```python
from build123d import *


with BuildPart() as part:
    # Sketch1 → Revolve1 (revolve)
    with BuildSketch(Plane.XY, mode=Mode.PRIVATE) as revolve1_sk:
        with BuildLine():
            Line((-40, 5), (-40, -15))
            ThreePointArc((-40, -15), (-38.535533906, -18.535533906), (-35, -20))
            Line((-35, -20), (-16, -20))
            ThreePointArc((-16, -20), (-11.757359313, -21.757359313), (-10, -26))
            Line((-10, -26), (-10, -28.486287513))
            Line((-10, -28.486287513), (-5.75, -28.486287513))
            Line((-5.75, -28.486287513), (-5.75, -22))
            ThreePointArc((-5.75, -22), (-7.507359313, -17.757359313), (-11.75, -16))
            Line((-11.75, -16), (-30, -16))
            ThreePointArc((-30, -16), (-33.535533906, -14.535533906), (-35, -11))
            Line((-35, -11), (-35, 10))
            Line((-35, 10), (-37.5, 10))
            Line((-37.5, 10), (-37.5, 5))
            Line((-37.5, 5), (-40, 5))
        make_face()
    revolve(revolve1_sk.sketch.rotate(Axis((0, 0, 0), (0, 1, 0)), 270), axis=Axis((0, 0, 0), (0, 1, 0)))


solid = part.part
```
Can you work these out from the model? Positions are in its coordinate system, mm. A direction names the side the tool comes from. Coordinates: 2 decimals unless noted, no trailing zeros. Write each loop counter-clockwise with the first axis right and the second up, starting at its lowest first coordinate (ties: lowest second). Pieces come first, ordered by that corner, then holes. Notation, with made-up numbers: M 1,-20.5 L 45,-20.5 A16 cw 45,2.5 Z; hole C 18,33.25 d9. An arc over 180 degrees is marked long. Write item = value, one per line. Start each with the question number.
Q1. On a 3-axis mill with a long thin cutter (end or side, diameter ignored), from which of +Z, -Z, +X, -X, +Y, -Y can I reach the whole of each face in a straight line? I mean faces 1 (the face through (9.76, -27.26, 2.17)), 2 (the face through (13, -16, 0)), 3 (the face through (4.3, -28.486, -4.3)). Say none if no direction works.
Q2. Thinking about a two-plate mould opening in X: for faces 4 (the face through (22.818, 7.465, 29.759)), 5 (the face through (-4.85, -25.2, -3.09)), 6 (the face through (-36, 5, 12)), which applies, released by +X, released by -X, zero draft, split by the parting line, or undercut?
Q3. If I drill on L1, parallel to X at y = 5.25, z = 0; L2, parallel to X at y = -3, z = 0; L3, parallel to Y at x = -15, z = -18.5, over which ranges is the centre line in solid material (lowest first)? Write a range as [from, to].
Q4. If we section it at A-A, the plane z = 0: Write out the boundary of the cut face in (x, y), then the cut area to 3 significant figures.
Q5. If we section it at B-B, the plane x = 0: Write out the boundary of the cut face in (y, z), then the cut area to 3 significant figures.
Q6. If we section it at C-C, the plane y = -4: Write out the boundary of the cut face in (x, z), then the cut area to 3 significant figures.
Q7. I'm going to push flat-ended pins straight in: pin 1 (6 mm diameter, centred on y = 0, z = -11, fed in from +X); pin 2 (8 mm diameter, centred on y = -5.5, z = -27, fed in from +X); pin 3 (6 mm diameter, centred on x = 8.5, y = -1.5, fed in from +Z). Where does each tip first touch, or does it pass through?
Check sheet entries:
q1.face_1 = -Y
q1.face_2 = +Y
q1.face_3 = +Z, -Z, +X, -X, -Y
q2.face_4 = split by the parting line
q2.face_5 = undercut
q2.face_6 = zero draft
q3.L1 = [-37.5, -35], [35, 37.5]
q3.L2 = [-40, -35], [35, 40]
q3.L3 = [-20, -16]
q4.outline = M -40,-15 A5 ccw -35,-20 L -16,-20 A6 cw -10,-26 L -10,-28.49 L -5.75,-28.49 L -5.75,-22 A6 ccw -11.75,-16 L -30,-16 A5 cw -35,-11 L -35,10 L -37.5,10 L -37.5,5 L -40,5 Z; M 5.75,-28.49 L 10,-28.49 L 10,-26 A6 cw 16,-20 L 35,-20 A5 ccw 40,-15 L 40,5 L 37.5,5 L 37.5,10 L 35,10 L 35,-11 A5 cw 30,-16 L 11.75,-16 A6 ccw 5.75,-22 Z
q4.area = 581 mm²
q5.outline = M -28.49,-10 L -26,-10 A6 cw -20,-16 L -20,-35 A5 ccw -15,-40 L 5,-40 L 5,-37.5 L 10,-37.5 L 10,-35 L -11,-35 A5 cw -16,-30 L -16,-11.75 A6 ccw -22,-5.75 L -28.49,-5.75 Z; M -28.49,5.75 L -22,5.75 A6 ccw -16,11.75 L -16,30 A5 cw -11,35 L 10,35 L 10,37.5 L 5,37.5 L 5,40 L -15,40 A5 ccw -20,35 L -20,16 A6 cw -26,10 L -28.49,10 Z
q5.area = 581 mm²
q6.outline = C 0,0 d80; hole C 0,0 d70
q6.area = 1,180 mm²
q7.pin_1 = 39.19
q7.pin_2 = 32.73
q7.pin_3 = 39.62
